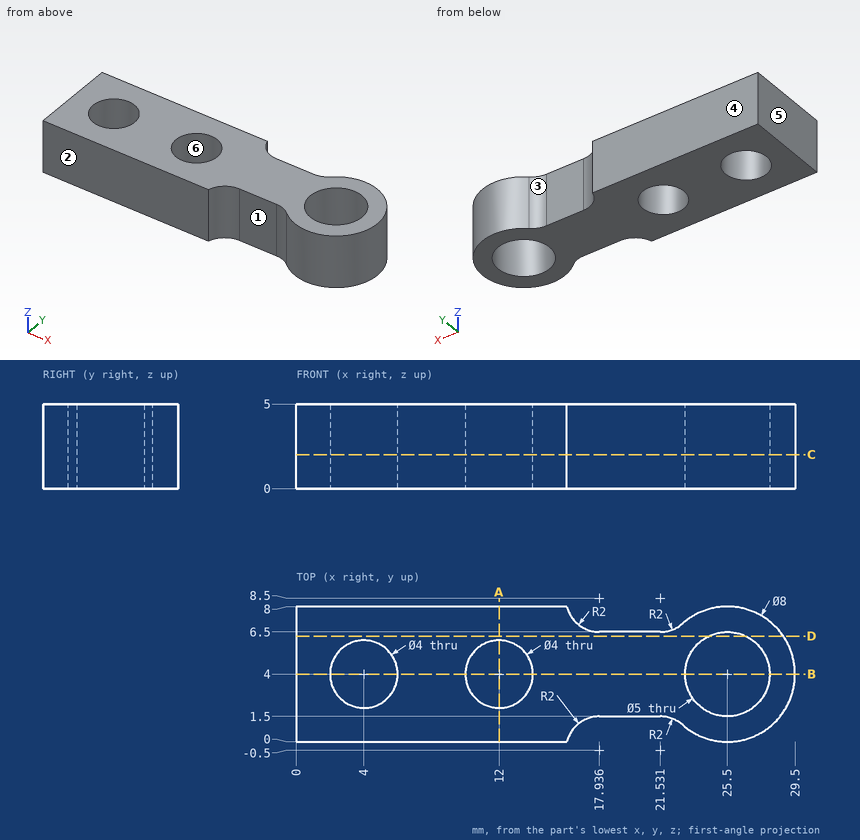
For this review, use the dimensioned drawing (mm, ordinates from the lowest corner) and the shaded views. A direction names the side the tool comes from. Give positions to 0.01 mm unless a question says otherwise; leave off trailing zeros. Order: outer loops, then holes, each group sorted by start corner. A loop starts at its lowest first (then second) coordinate and runs counter-clockwise, first axis right, second up. Notation, with made-up numbers: (52.5, -20) - (80.5, -20) arc R26 cw to (80.5, 4) - close; hole circle Ø10 at (-16.5, 24.25). An arc over 180 degrees is marked (long way). Use a Markdown table: item, result. Add a question column.
(1) Wall thickness on probe 1 along Y at (x, z) = (25.5, 1.1); probe 2 along Y at (x, z) = (4, 2.2); probe 3 along X at (y, z) = (5.5, 1) (1 decimal): over which ranges is each line inside the solid? List them lowest first. Write a range as [from, to].
(2) Machinability: for the marked faces 1, 2 and 3, which of the approach directions +Z, -Z, +X, -X, +Y, -Y give a long, thin tool a straight path to every point of the face, cutting with its end or side? Answer none if there is none.
(3) Add section C-C on z = 2. Give the boundary of the cut face in (x, y) (1 decimal), then the cut area to 3 significant figures.
(4) Add section D-D on y = 6.25. Give the boundary of the cut face in (x, z).
(5) Mouldability with a two-part tool opening along X and no side actions: class the marked faces 4, 5 and 6 as +X half, -X half, draft (parallel to the pull), parting line (faces both ways), or undercut.
(6) Add section B-B on y = 4. Give the boundary of the cut face in (x, z).
(7) Clearance check with flat-ended pins moving along their axes: P1, Ø1.8, axis at x = 20.5, z = 2, coming from the +Y side; P2, Ø3, axis at x = 19.5, z = 3.5, coming from the -Y side. State where each tip first meets the part, or that it passes through.
(8) Add section A-A on x = 12. Give the boundary of the cut face in (y, z), then the cut area to 3 significant figures.
Report:
| question | item | result |
|---|---|---|
| 1 | probe 1 | y = [0, 1.5], [6.5, 8] |
| 1 | probe 2 | y = [0, 2], [6, 8] |
| 1 | probe 3 | x = [0, 2.7], [5.3, 10.7], [13.3, 23.5], [27.5, 29.2] |
| 2 | face 1 | +Z, -Z, -Y |
| 2 | face 2 | +Z, -Z, +X, -X, -Y |
| 2 | face 3 | +Z, -Z, +Y |
| 3 | outline | (0, 0) - (16, 0) arc R2 cw to (17.9, 1.5) - (21.5, 1.5) arc R2 cw to (22.9, 1) arc R4 ccw (long way) to (22.9, 7) arc R2 cw to (21.5, 6.5) - (17.9, 6.5) arc R2 cw to (16, 8) - (0, 8) - close; hole circle Ø4 at (4, 4); hole circle Ø4 at (12, 4); hole circle Ø5 at (25.5, 4) |
| 3 | area | 164 mm² |
| 4 | outline | (0, 0) - (24.41, 0) - (24.41, 5) - (0, 5) - close; (26.59, 0) - (28.81, 0) - (28.81, 5) - (26.59, 5) - close |
| 5 | face 4 | draft |
| 5 | face 5 | -X half |
| 5 | face 6 | undercut |
| 6 | outline | (0, 0) - (2, 0) - (2, 5) - (0, 5) - close; (6, 0) - (10, 0) - (10, 5) - (6, 5) - close; (14, 0) - (23, 0) - (23, 5) - (14, 5) - close; (28, 0) - (29.5, 0) - (29.5, 5) - (28, 5) - close |
| 7 | P1 | stops at y = 6.5 |
| 7 | P2 | stops at y = 1.5 |
| 8 | outline | (0, 0) - (2, 0) - (2, 5) - (0, 5) - close; (6, 0) - (8, 0) - (8, 5) - (6, 5) - close |
| 8 | area | 20.0 mm² |
